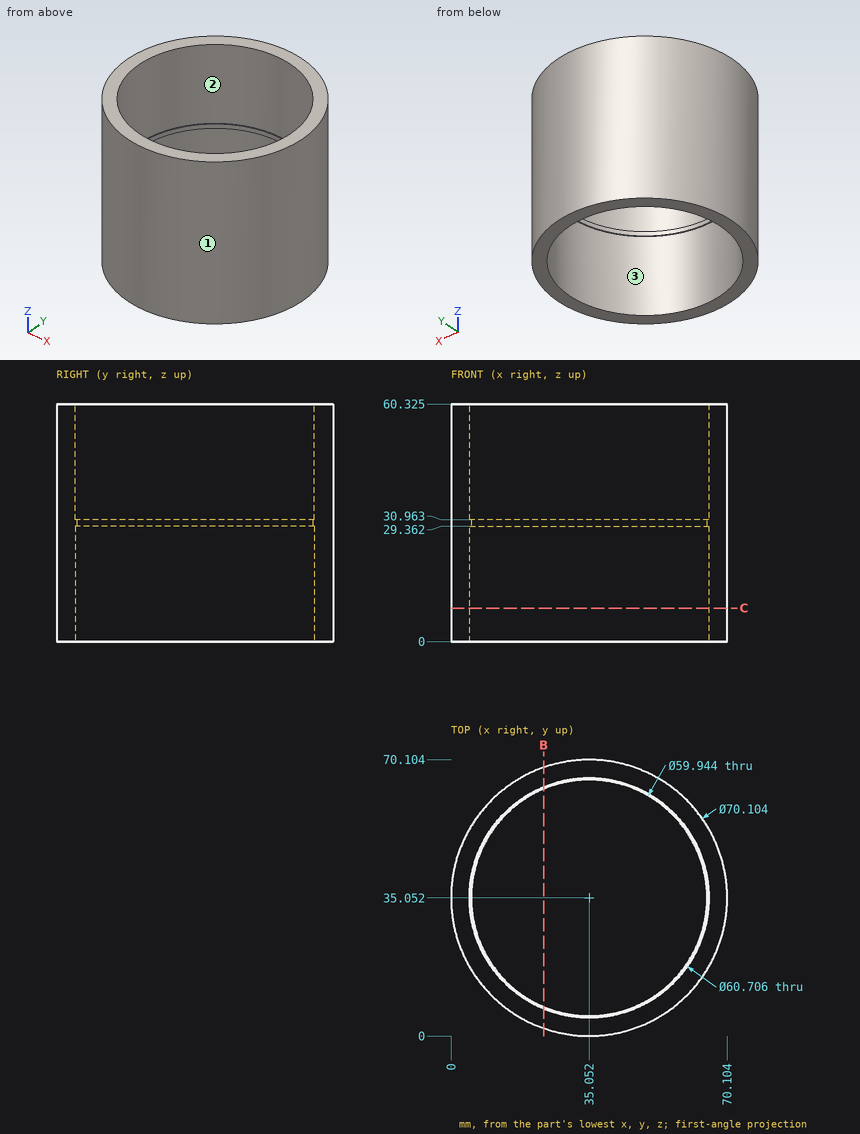
Geometry: see drawing. Coordinates: mm, zero at the bounding-box minimum. Give positions to 0.01 mm unless a question says otherwise; leave off trailing zeros. Order: outer loops, then holes, each group sorted by start corner. A loop starts at its lowest first (then second) coordinate and runs counter-clockwise, first axis right, second up.
1. Line query: probe 1 along X at (y, z) = (50, 31) (1 decimal); probe 2 along Y at (x, z) = (25, 6); probe 3 along Y at (x, z) = (32, 54.5). Output: solid intervals per line, ascending.
Computed:
probe 1: x = 3.3 to 8.6, 61.5 to 66.8
probe 2: y = 1.47 to 6.41, 63.69 to 68.63
probe 3: y = 0.13 to 4.85, 65.25 to 69.97
2. Cut plane B-B (x = 23.5). Return loops of the section in (y, z) (1 decimal).
Computed:
outline: (2, 0) - (7, 0) - (7, 29.4) - (7.4, 29.4) - (7.4, 31) - (7, 31) - (7, 60.3) - (2, 60.3) - close; (62.7, 29.4) - (63.1, 29.4) - (63.1, 0) - (68.1, 0) - (68.1, 60.3) - (63.1, 60.3) - (63.1, 31) - (62.7, 31) - close
3. Cut plane C-C (z = 8.5). Return loops of the section in (x, y).
Computed:
outline: circle Ø70.1 at (35.05, 35.05); hole circle Ø60.71 at (35.05, 35.05)
4. Draft query along Y for the marked faces 1, 2 and 3. Return one class per face: released by +Y, released by -Y, zero draft, split by the parting line, or undercut.
Computed:
face 1: split by the parting line
face 2: undercut
face 3: undercut
5. Pin query (flat end, axial travel): pin 1 Ø4 at (y, z) = (46.5, 9) entering from +X; pin 2 Ø4 at (y, z) = (31.5, 12.5) entering from +X; pin 3 Ø12 at (x, z) = (23, 27.5) entering from -Y. Return the tip coordinate at first contact, or that it passes through.
Computed:
pin 1: stops at x = 68.81
pin 2: stops at x = 70.07
pin 3: stops at y = 0.53
